```python
from build123d import *

# Parameters (mm, degrees)
F1_DEPTH        = 1050.925
F2_W            = 273.05
F2_H            = 368.808
F3_DEPTH        = 3.175
F5_D            = 14.224
F5_DEPTH        = 31.75
F5_CBORE_D      = 28.575
F5_CBORE_DEPTH  = 3.175
F5_TIP          = 4.2733207225
F6_W            = 304.8
F6_H            = 31.75
F7_DEPTH        = 25.4
F8_R            = 15.875
F9_W            = 304.8
F9_H            = 374.65
F10_DEPTH       = 44.45
F12_D           = 27.0002
F12_CBORE_D     = 53.975
F12_CBORE_DEPTH = 3.175
F15_DEPTH       = 76.2
F17_D           = 38.89248
F18_W           = 76.2
F18_H           = 25.4
F19_DEPTH       = 12.7


with BuildPart() as f1:
    # F0 (on Right) → F1 (new body)
    with BuildSketch(Plane.YZ):
        with BuildLine():
            Line((184.404, 178.054), (-184.404, 178.054))
            Line((-184.404, 178.054), (-184.404, 160.02))
            Line((-184.404, 160.02), (-23.368, 160.02))
            ThreePointArc((-23.368, 160.02), (-10.7956414305, 154.8123585695), (-5.588, 142.24))
            Line((-5.588, 142.24), (-5.588, -142.24))
            ThreePointArc((-5.588, -142.24), (-10.7956414305, -154.8123585695), (-23.368, -160.02))
            Line((-23.368, -160.02), (-184.404, -160.02))
            Line((-184.404, -160.02), (-184.404, -178.054))
            Line((-184.404, -178.054), (184.404, -178.054))
            Line((184.404, -178.054), (184.404, -160.02))
            Line((184.404, -160.02), (23.368, -160.02))
            ThreePointArc((23.368, -160.02), (10.7956414305, -154.8123585695), (5.588, -142.24))
            Line((5.588, -142.24), (5.588, 142.24))
            ThreePointArc((5.588, 142.24), (10.7956414305, 154.8123585695), (23.368, 160.02))
            Line((23.368, 160.02), (184.404, 160.02))
            Line((184.404, 160.02), (184.404, 178.054))
        make_face()
    extrude(amount=F1_DEPTH)

    # F2 (on face) → F3 (cut)
    with BuildSketch(Plane.XY.offset(178.054)):
        with Locations((901.7, 0)):
            Rectangle(F2_W, F2_H)
    extrude(amount=-F3_DEPTH, mode=Mode.SUBTRACT)

    # F5
    with Locations(Plane.XY.offset(174.879)):
        with Locations((793.623, 101.6), (1009.523, 101.6), (793.623, -101.6), (1009.523, -101.6)):
            CounterBoreHole(F5_D / 2, F5_CBORE_D / 2, F5_CBORE_DEPTH, depth=F5_DEPTH)
            with Locations((0, 0, -(F5_DEPTH + F5_TIP / 2))):  # 118° drill point
                Cone(0, F5_D / 2, F5_TIP, mode=Mode.SUBTRACT)

    # F6 (on face) → F7 (cut)
    with BuildSketch(Plane.XY.offset(178.054)):
        with Locations((898.525, 168.529)):
            Rectangle(F6_W, F6_H)
        with Locations((898.525, -168.529)):
            Rectangle(F6_W, F6_H)
    extrude(amount=-F7_DEPTH, mode=Mode.SUBTRACT)

    # F8
    f8_edges = [f1.edges().sort_by_distance(p)[0] for p in [
        (746.125, -152.654, 169.037),
        (746.125, 152.654, 169.037),
    ]]
    fillet(f8_edges, radius=F8_R)

    # F9 (on face) → F10 (join)
    with BuildSketch(Plane.YZ.offset(1050.925)):
        Rectangle(F9_W, F9_H)
    extrude(amount=F10_DEPTH)

    # F12 (through all)
    with Locations(Plane(origin=(1050.925, 0, 0), x_dir=(0, -1, 0), z_dir=(-1, 0, 0))):
        with Locations((-114.3, 101.854), (-114.3, -114.046), (114.3, 101.854), (114.3, -114.046)):
            CounterBoreHole(F12_D / 2, F12_CBORE_D / 2, F12_CBORE_DEPTH)

    # F14 (on offset) → F15 (join)
    with BuildSketch(Plane.YZ.offset(939.673)):
        Polygon((-5.588, -142.24), (-5.588, 119.38), (-211.074, 119.38), (-323.088, 231.394), (-475.488, 231.394), (-475.488, 131.064), (-184.404, -160.02), (-23.368, -160.02), align=None)
    extrude(amount=-F15_DEPTH)

    # F17 (through all)
    with Locations(Plane.XY.offset(231.394)):
        with Locations((901.573, -425.45)):
            Hole(F17_D / 2)

    # F18 (on face) → F19 (cut)
    with BuildSketch(Plane.XY.offset(231.394)):
        with Locations((901.573, -385.7752)):
            Rectangle(F18_W, F18_H)
    extrude(amount=-F19_DEPTH, mode=Mode.SUBTRACT)

    # F20: F1 across plane


with BuildPart() as f1_1:
    add(f1.part)
    add(f1.part.mirror(Plane.YZ))


solid = f1_1.part
```
Geometry: final body of the model. Coordinates: model frame, mm. A direction names the side the tool comes from. Round coordinates to 2 decimals unless told otherwise and drop trailing zeros. Order: outer loops, then holes, each group sorted by start corner. A loop starts at its lowest first (then second) coordinate and runs counter-clockwise, first axis right, second up. Notation, with made-up numbers: (21.25, -15) -> (69.25, -15) arc R24 ccw to (69.25, 15) -> close; hole circle Ø7 at (-19, -40). An arc over 180 degrees is marked (long way). Use CSV: the item, a comma, the result in double quotes. Start each with the question number.
1) Section C-C (z = -11.5). Return the cut outline in (x, y) (3 decimals), and give its area (3 significant figures).
2) Section D-D (y = -259). Return the cut outline in (x, z).
3) First-contact query: pin 1 Ø1.5 at (x, z) = (-171, 141) entering from +Y; pin 2 Ø12 at (y, z) = (-299, 63) entering from -X; pin 3 Ø9 at (y, z) = (-171.5, -168.5) entering from -X (3 decimals). Flat tips, straight axial feed; report the tip coordinate or a pass-through.
4) Set-up query: faces 1 (the face through (1054.1, 127, 96)), 2 (the face through (1073, -152.4, -3)), 3 (the face through (1050.925, -80, 2)), 4 (the face through (902.106, -266.297, 174.603)). Return all of +Z, -Z, +X, -X, +Y, -Y with unobstructed straight access to the full face (end or side cutting, diameter ignored); none if empty.
5) Material intervals for line 1 along Z through (x, y) = (-1064, 114.3) (3 decimals); line 2 along Z through (x, y) = (-1052, 114) (3 decimals); line 3 along X through (y, z) = (-32, 67) (3 decimals), sorted ascending. Write a range as from..to.
6) Section B-B (y = -425.45). Return the cut outline in (x, z).
7) Draft query along Z for faces 5 (the face through (1073, -2, -187.325)), 6 (the face through (904.1, -406.17, 145.3)), 7 (the face through (-902, -107, 119.38)), 8 (the face through (-1052.49, -108.45, 75.51)). Return one class per face: +Z half, -Z half, draft (parallel to the pull), parting line (faces both ways), or undercut.
8) Section A-A (x = -219). Return the cut outline in (y, z), and give its area (3 significant figures).
Returned:
1,outline,"(-1095.375, -152.4) -> (-1050.925, -152.4) -> (-1050.925, -5.588) -> (-939.673, -5.588) -> (-939.673, -332.924) -> (-863.473, -332.924) -> (-863.473, -5.588) -> (863.473, -5.588) -> (863.473, -332.924) -> (939.673, -332.924) -> (939.673, -5.588) -> (1050.925, -5.588) -> (1050.925, -152.4) -> (1095.375, -152.4) -> (1095.375, 152.4) -> (1050.925, 152.4) -> (1050.925, 5.588) -> (-1050.925, 5.588) -> (-1050.925, 152.4) -> (-1095.375, 152.4) -> close"
1,area,"100,000 mm²"
2,outline,"(-939.67, -85.42) -> (-863.47, -85.42) -> (-863.47, 167.31) -> (-939.67, 167.31) -> close; (863.47, -85.42) -> (939.67, -85.42) -> (939.67, 167.31) -> (863.47, 167.31) -> close"
3,pin 1,"stops at y = 5.59"
3,pin 2,"stops at x = -939.67"
3,pin 3,"stops at x = -1050.925"
4,face 1,"none"
4,face 2,"+Z, -Z, +X, -Y"
4,face 3,"-Y"
4,face 4,"+Z, +X, -X"
5,line 1,"z = -187.325..-127.546, -100.546..88.354, 115.354..187.325"
5,line 2,"z = -187.325..-141.032, -87.06..74.868, 128.84..187.325"
5,line 3,"x = -1095.375..-1050.925, -939.673..-863.473, 863.473..939.673, 1050.925..1095.375"
6,outline,"(-939.67, 81.03) -> (-921.02, 81.03) -> (-921.02, 231.39) -> (-939.67, 231.39) -> close; (-882.13, 81.03) -> (-863.47, 81.03) -> (-863.47, 231.39) -> (-882.13, 231.39) -> close; (863.47, 81.03) -> (882.13, 81.03) -> (882.13, 231.39) -> (863.47, 231.39) -> close; (921.02, 81.03) -> (939.67, 81.03) -> (939.67, 231.39) -> (921.02, 231.39) -> close"
7,face 5,"-Z half"
7,face 6,"draft"
7,face 7,"undercut"
7,face 8,"undercut"
8,outline,"(-184.4, -178.05) -> (184.4, -178.05) -> (184.4, -160.02) -> (23.37, -160.02) arc R17.78 cw to (5.59, -142.24) -> (5.59, 142.24) arc R17.78 cw to (23.37, 160.02) -> (184.4, 160.02) -> (184.4, 178.05) -> (-184.4, 178.05) -> (-184.4, 160.02) -> (-23.37, 160.02) arc R17.78 cw to (-5.59, 142.24) -> (-5.59, -142.24) arc R17.78 cw to (-23.37, -160.02) -> (-184.4, -160.02) -> close"
8,area,"17,200 mm²"
